from build123d import *

# Parameters (mm, degrees)
SKETCH_1_R      = 3
SKETCH_1_R_2    = 1.5
EXTRUDE_1_DEPTH = 6
SKETCH_2_R      = 2.25
SKETCH_2_R_2    = 1.5
EXTRUDE_2_DEPTH = 8
SKETCH_3_R      = 3
SKETCH_3_R_2    = 1.5
EXTRUDE_3_DEPTH = 6
CHAMFER_1_SIZE  = 0.8
FILLET_1_R      = 0.1


with BuildPart() as part:
    # 草图1 → 凸台-拉伸1 (new body)
    with BuildSketch(Plane(origin=(0, 0, 0), x_dir=(1, 0, 0), z_dir=(0, 1, 0))):
        with Locations(Location((0, 0, 0), (0, 0, 270))):
            Circle(SKETCH_1_R)
        with Locations(Location((0, 0, 0), (0, 0, 270))):
            Circle(SKETCH_1_R_2, mode=Mode.SUBTRACT)
    extrude(amount=EXTRUDE_1_DEPTH)

    # 草图2 → 凸台-拉伸2 (add)
    with BuildSketch(Plane(origin=(0, 6, 0), x_dir=(1, 0, 0), z_dir=(0, 1, 0))):
        with Locations(Location((0, 0, 0), (0, 0, 270))):
            Circle(SKETCH_2_R)
        with Locations(Location((0, 0, 0), (0, 0, 270))):
            Circle(SKETCH_2_R_2, mode=Mode.SUBTRACT)
    extrude(amount=EXTRUDE_2_DEPTH)

    # 草图3 → 凸台-拉伸3 (add)
    with BuildSketch(Plane(origin=(0, 14, 0), x_dir=(1, 0, 0), z_dir=(0, 1, 0))):
        with Locations(Location((0, 0, 0), (0, 0, 270))):
            Circle(SKETCH_3_R)
        with Locations(Location((0, 0, 0), (0, 0, 270))):
            Circle(SKETCH_3_R_2, mode=Mode.SUBTRACT)
    extrude(amount=EXTRUDE_3_DEPTH)

    # 倒角1
    # the kernel refuses this chamfer: 0.8 mm, written as the material it takes off along each edge
    with BuildSketch(Plane(origin=(0, 6, 0), x_dir=(0, 0, 1), z_dir=(-1, 0, 0))) as chamfer_1_piece_1_section:
        Polygon((3, -CHAMFER_1_SIZE), (3 - CHAMFER_1_SIZE, 0), (3, 0), align=None)
    chamfer_1_piece_1 = revolve(axis=Axis((0, 6, 0), (0, 1, 0)), mode=Mode.PRIVATE)
    chamfer_1_piece_1 = chamfer_1_piece_1 - Plane(origin=(0, 5.57653803, 0), x_dir=(0, 0, 1), z_dir=(0, -1, 0)) * Cylinder(2.25, 12, mode=Mode.PRIVATE)
    add(chamfer_1_piece_1, mode=Mode.SUBTRACT)
    with BuildSketch(Plane(origin=(0, 14, 0), x_dir=(0, 0, 1), z_dir=(-1, 0, 0))) as chamfer_1_piece_2_section:
        Polygon((3 - CHAMFER_1_SIZE, 0), (3, CHAMFER_1_SIZE), (3, 0), align=None)
    chamfer_1_piece_2 = revolve(axis=Axis((0, 14, 0), (0, 1, 0)), mode=Mode.PRIVATE)
    chamfer_1_piece_2 = chamfer_1_piece_2 - Plane(origin=(0, 14.42346197, 0), x_dir=(0, 0, 1), z_dir=(0, -1, 0)) * Cylinder(2.25, 13, mode=Mode.PRIVATE)
    add(chamfer_1_piece_2, mode=Mode.SUBTRACT)

    # 圆角1
    fillet_1_edges = [part.edges().sort_by_distance(p)[0] for p in [
        (0, 20, -3),
        (0, 0, -3),
        (0, 5.2, -3),
        (0, 14.8, -3),
    ]]
    fillet(fillet_1_edges, radius=FILLET_1_R)


solid = part.part
Verification items for the finished model (mm, model axes). Round coordinates to 2 decimals unless told otherwise and drop trailing zeros. Loops run counter-clockwise (first coordinate to the right, second up) from the corner with the lowest first, then second, coordinate; pieces in that order, holes last. Notation, with made-up numbers: (42.25, 75) - (56.25, 75) arc R18 cw to (56.25, 85) - close; hole circle Ø4 at (42.25, -39.5). An arc over 180 degrees is marked (long way). Write item = value, one per line.
Q1. Mould release check, pull along Z, two halves, no side actions. Record for faces 1 (the flat face through (-1.2, 20, 1.2)), 2 (the cylindrical face through (-1.15, 2.59, 2.77)), 3 (the cylindrical face through (0.45, 9.86, 1.43)): +Z half, -Z half, draft (parallel to the pull), parting line (faces both ways), or undercut.
Here are the results:
face_1 = draft
face_2 = parting line
face_3 = undercut
Q2. Sectioned sample at A-A on y = 13.25. Record the boundary of the cut face in (x, z).
Here are the results:
outline = circle Ø4.5 at (0, 0); hole circle Ø3 at (0, 0)
Q3. Depth check by flat-ended pin: pin 1 (1.5 mm diameter, centred on y = 14, z = 0.5, fed in from -X); pin 2 (1 mm diameter, centred on x = -1, z = 1, fed in from -Y); pin 3 (1 mm diameter, centred on y = 14, z = 2, fed in from -X); pin 4 (1.5 mm diameter, centred on x = 1, y = 16, fed in from -Z). Enter the tip coordinate at first touch or a pass-through.
Here are the results:
pin_1 = -2.92
pin_2 = 0
pin_3 = -1.97
pin_4 = -2.99
Q4. Material ranges on L1, parallel to X at y = 6.5, z = 0; L2, parallel to X at y = 15, z = 0; L3, parallel to Y at x = -2.5, z = 0.5, recorded low to high.
Here are the results:
L1 = -2.25 to -1.5, 1.5 to 2.25
L2 = -3 to -1.5, 1.5 to 3
L3 = 0 to 5.65, 14.35 to 20
